from build123d import *

# Parameters (mm, degrees)
EXTRUDE_1_DEPTH          = 10.5
EXTRUDE_1_DEPTH_BACK     = 10.5
SKETCH_1_W               = 25.3
SKETCH_1_H               = 16
EXTRUDE_2_DEPTH          = 12.6
EXTRUDE_2_DEPTH_BACK     = 12.6
SKETCH_2_W               = 31
SKETCH_2_H               = 2.1
EXTRUDE_3_DEPTH          = 9.2
EXTRUDE_3_DEPTH_BACK     = 9.2
EXTRUDE_4_DEPTH          = 8.3
EXTRUDE_4_DEPTH_BACK     = 8.3
SKETCH_5_W               = 1
SKETCH_5_H               = 6.1
EXTRUDE_5_DEPTH          = 9
SKETCH_6_W               = 25.3
SKETCH_6_H               = 1.1
EXTRUDE_6_DEPTH          = 8
CUT_EXTRUDE_1_DEPTH      = 38.866773034
CUT_EXTRUDE_1_DEPTH_BACK = 38.866773034
SKETCH_7_R               = 1.5
SKETCH_7_R_2             = 1.3


with BuildPart() as part:
    # 草图1 → 凸台-拉伸1 (new, two sides: drawn at the far end of the back side and taken through both)
    with BuildSketch(Plane.XY.offset(-EXTRUDE_1_DEPTH_BACK)):
        with Locations((12.65, 8)):
            Rectangle(SKETCH_1_W, SKETCH_1_H)
    extrude(amount=EXTRUDE_1_DEPTH + EXTRUDE_1_DEPTH_BACK)

    # 草图2 → 凸台-拉伸2 (add, two sides: drawn at the far end of the back side and taken through both)
    with BuildSketch(Plane.XY.offset(-EXTRUDE_2_DEPTH_BACK)):
        with Locations((12.65, 17.05)):
            Rectangle(SKETCH_2_W, SKETCH_2_H)
    extrude(amount=EXTRUDE_2_DEPTH + EXTRUDE_2_DEPTH_BACK)

    # 草图3 → 凸台-拉伸3 (add, two sides: drawn at the far end of the back side and taken through both)
    with BuildSketch(Plane.XY.offset(-EXTRUDE_3_DEPTH_BACK)):
        with BuildLine():
            Line((1.4, 18.1), (23.9, 18.1))
            ThreePointArc((23.9, 18.1), (14.246241567, 19.638076247), (5.548427655, 24.1))
            ThreePointArc((5.548427655, 24.1), (2.206514702, 21.976493018), (1.4, 18.1))
        make_face()
    extrude(amount=EXTRUDE_3_DEPTH + EXTRUDE_3_DEPTH_BACK)

    # 草图4 → 凸台-拉伸4 (add, two sides: drawn at the far end of the back side and taken through both)
    with BuildSketch(Plane.XY.offset(-EXTRUDE_4_DEPTH_BACK)):
        Polygon((0, 0), (-2.85, 12.5), (-1.85, 15.8), (-0.805094567, 15.8), (-0.892975596, 15.509992605), (-1.816075348, 12.463763423), (0, 4.498520669), align=None)
        Polygon((25.3, 0), (25.3, 4.498520669), (27.116075348, 12.463763423), (26.192975596, 15.509992605), (26.105094567, 15.8), (27.15, 15.8), (28.15, 12.5), align=None)
    extrude(amount=EXTRUDE_4_DEPTH + EXTRUDE_4_DEPTH_BACK)

    # 草图5 → 凸台-拉伸5 (add)
    with BuildSketch(Plane.XZ):
        with Locations((23, -5.25)):
            Rectangle(SKETCH_5_W, SKETCH_5_H)
        with Locations((12.65, -5.25)):
            Rectangle(SKETCH_5_W, SKETCH_5_H)
        with Locations((2.3, -5.25)):
            Rectangle(SKETCH_5_W, SKETCH_5_H)
        with Locations((2.3, 5.25)):
            Rectangle(SKETCH_5_W, SKETCH_5_H)
        with Locations((12.65, 5.25)):
            Rectangle(SKETCH_5_W, SKETCH_5_H)
        with Locations((23, 5.25)):
            Rectangle(SKETCH_5_W, SKETCH_5_H)
    extrude(amount=EXTRUDE_5_DEPTH)

    # 草图6 → 凸台-拉伸6 (add)
    with BuildSketch(Plane.XZ):
        with Locations((12.65, 0)):
            Rectangle(SKETCH_6_W, SKETCH_6_H)
    extrude(amount=EXTRUDE_6_DEPTH)

    # 草图7 → 切除-拉伸1 (cut, two sides: drawn at the far end of the back side and taken through both)
    with BuildSketch(Plane(origin=(23.5, 0, 0), x_dir=(0, 0, -1), z_dir=(1, 0, 0)).offset(-CUT_EXTRUDE_1_DEPTH_BACK)):
        with Locations((-5.106619867, -6)):
            Circle(SKETCH_7_R)
        with Locations((-5.106619867, -1.714294339)):
            Circle(SKETCH_7_R_2)
        Polygon((-6.8, -9), (-8.3, -7.5), (-8.3, -9), align=None)
        Polygon((2.2, -7.5), (2.2, -9), (3.697628314, -9), align=None)
        Polygon((-2.2, -7.5), (-3.697628314, -9), (-2.2, -9), align=None)
        Polygon((8.3, -7.5), (6.8, -9), (8.3, -9), align=None)
        with Locations((5.106619867, -6)):
            Circle(SKETCH_7_R)
        with Locations((5.106619867, -1.714294339)):
            Circle(SKETCH_7_R_2)
    extrude(amount=CUT_EXTRUDE_1_DEPTH + CUT_EXTRUDE_1_DEPTH_BACK, mode=Mode.SUBTRACT)


solid = part.part
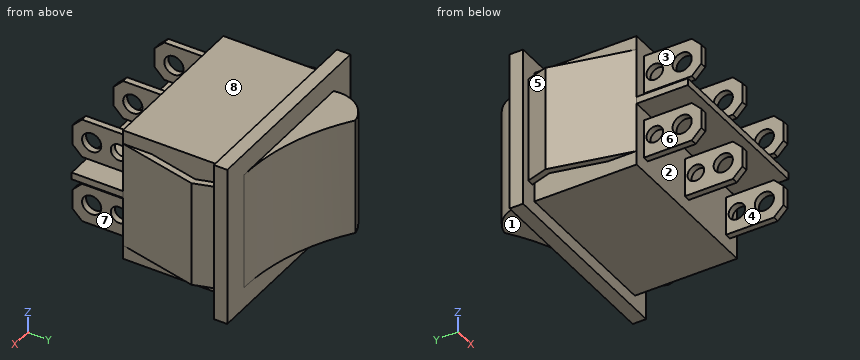
Geometry: final body of the model. Coordinates: model frame, mm. Face numbers are marked on the shaded views. A direction names the side the tool comes from. Round coordinates to 2 decimals unless told otherwise and drop trailing zeros. Loops run counter-clockwise (first coordinate to the right, second up) from the corner with the lowest first, then second, coordinate; pieces in that order, holes last. Notation, with made-up numbers: M -27.75,50 L 7.25,50 A21 cw 7.25,60 Z; hole C -9,86.5 d8. An arc over 180 degrees is marked long. Put each result on its own line as item: value. Start each with the question number.
(1) Section query D-D (y = 20). Return loops of the section in (x, z).
(2) Section query B-B (y = -6). State how many separate pieces and enclosed holes the cut face has, then the cut area to 3 significant figures.
(3) Draft query along X for the marked faces 1, 2, 3 and 4. Return one class per face: +X half, -X half, draft (parallel to the pull), parting line (faces both ways), or undercut.
(4) Contact query for flat-ended pins moving along their axis: pin 1 Ø5 at (y, z) = (-4, -6) entering from -X; pin 2 Ø1 at (x, y) = (15, 8) entering from +Z; pin 3 Ø8 at (x, y) = (24, -2.5) entering from -Z. Output: stop coordinate, or through.
(5) Section query A-A (y = 5). Return loops of the section in (x, z).
(6) Material intervals for line 1 along Z through (x, y) = (23.3, -6); line 2 along X through (y, z) = (6.5, 5); line 3 along X through (y, z) = (7, -2.75), sorted ascending. Write a range as [from, to].
(7) Set-up query: the marked faces 5, 6, 7 and 8. Return all of +Z, -Z, +X, -X, +Y, -Y with unobstructed straight access to the full face (end or side cutting, diameter ignored); none if empty.
(8) Section query C-C (x = 20.5). Return loops of the section in (y, z).
Findings below:
1. outline: M 1.39,-9.2 L 13.2,-9.2 L 13.2,9.2 L 1.39,9.2 Z
2. separate pieces: 13
2. enclosed holes: 0
2. area: 46.4 mm2
3. face 1: draft
3. face 2: undercut
3. face 3: -X half
3. face 4: undercut
4. pin 1: stops at x = 1.8
4. pin 2: stops at z = 10.5
4. pin 3: stops at z = -10.5
5. outline: M -1.14,-8.3 L -0.11,-8.3 L -0.11,8.3 L -1.14,8.3 Z; M 0,-10.5 L 25.3,-10.5 L 25.3,10.5 L 0,10.5 Z; M 25.41,-8.3 L 26.44,-8.3 L 26.44,8.3 L 25.41,8.3 Z
6. line 1: z = [-8.3, -6.61], [-3.61, -2.2], [-0.55, 0.55], [2.2, 3.61], [6.61, 8.3]
6. line 2: x = [-1.48, -0.46], [0, 25.3], [25.76, 26.78]
6. line 3: x = [-1.6, -0.57], [0, 25.3], [25.87, 26.9]
7. face 5: +Z, -Z, -X
7. face 6: -Z, -X, -Y
7. face 7: -Z, +X, -Y
7. face 8: +Z, +X, -X, -Y
8. outline: M -8,-0.55 L 0,-0.55 L 0,-10.5 L 16,-10.5 L 16,-12.6 L 18.1,-12.6 L 18.1,-9.2 L 18.29,-9.2 L 18.29,9.2 L 18.1,9.2 L 18.1,12.6 L 16,12.6 L 16,10.5 L 0,10.5 L 0,0.55 L -8,0.55 Z
